Input: part model. Units: mm. Frame: model coordinates. Face numbers are marked on the shaded views. A direction names the side the tool comes from. Coordinates: 2 decimals unless noted, no trailing zeros. Order: outer loops, then holes, each group sorted by start corner. A loop starts at its lowest first (then second) coordinate and runs counter-clockwise, first axis right, second up. Notation, with made-up numbers: (56, 64.5) -> (109, 64.5) arc R34 ccw to (109, 94.5) -> close; hole circle Ø1 at (-8.75, -24.5). An arc over 180 degrees is marked (long way). Use one line per item in the form item = value. Start each with the question number.
1) Ray query, line 1 along X through (y, z) = (12.9, -96.25); line 2 along Z through (x, y) = (61.5, 12.5); line 3 along X through (y, z) = (12, -1). Return the intervals inside material, ascending.
2) Section query C-C on z = -77.5. Output: boundary loops of the cut face in (x, y), then the cut area to 3 significant figures.
3) Section query A-A on x = 36. Output: boundary loops of the cut face in (y, z), then the cut area to 3 significant figures.
4) Section query B-B on y = 15.5. Output: boundary loops of the cut face in (x, z), then the cut area to 3 significant figures.
5) Pin query (flat end, axial travel): pin 1 (1.2 mm diameter, centred on x = 59.5, y = 22.9, fed in from +Z); pin 2 (4 mm diameter, centred on y = 29, z = -70.5, fed in from -X); pin 3 (5 mm diameter, centred on x = 15, z = -66, fed in from +Y). Return the tip coordinate at first contact, or that it passes through.
6) Access query for the marked faces 1 and 2. Directions: +Z, -Z, +X, -X, +Y, -Y. A direction counts if a zero-diameter tool reaches every point of the face in a straight line with its end or side. Return the directions, or none.
from build123d import *

# Parameters (mm, degrees)
SKETCH1_W            = 70
SKETCH1_H            = 50
BOSS_EXTRUDE1_DEPTH  = 7.5
SKETCH2_W            = 70
SKETCH2_H            = 5
BOSS_EXTRUDE2_DEPTH  = 25
SKETCH3_R            = 1
SKETCH3_W            = 42
SKETCH3_H            = 21
CUT_EXTRUDE1_DEPTH   = 30
SKETCH27_W           = 5
SKETCH27_H           = 25
BOSS_EXTRUDE18_DEPTH = 45


with BuildPart() as part:
    # Sketch1 → Boss-Extrude1 (new body)
    with BuildSketch(Plane(origin=(0, 0, 0), x_dir=(1, 0, 0), z_dir=(0, 1, 0))):
        with Locations((35, 25)):
            Rectangle(SKETCH1_W, SKETCH1_H)
    boss_extrude1 = extrude(amount=BOSS_EXTRUDE1_DEPTH)

    # Sketch2 → Boss-Extrude2 (add)
    with BuildSketch(Plane(origin=(0, 7.5, 0), x_dir=(1, 0, 0), z_dir=(0, 1, 0))):
        with Locations((35, 2.5)):
            Rectangle(SKETCH2_W, SKETCH2_H)
    boss_extrude2 = extrude(amount=BOSS_EXTRUDE2_DEPTH)

    # Sketch3 → Cut-Extrude1 (cut)
    with BuildSketch(Plane.XY):
        with Locations((9.720773398, 22.9)):
            Circle(SKETCH3_R)
        with Locations((9.720773398, 12.9)):
            Circle(SKETCH3_R)
        with Locations((59.5, 12.9)):
            Circle(SKETCH3_R)
        with Locations((59.5, 22.9)):
            Circle(SKETCH3_R)
        with Locations((34.5, 18)):
            Rectangle(SKETCH3_W, SKETCH3_H)
    cut_extrude1 = extrude(amount=-CUT_EXTRUDE1_DEPTH, mode=Mode.SUBTRACT)

    # Sketch27 → Boss-Extrude18 (add)
    with BuildSketch(Plane(origin=(0, 0, -5), x_dir=(-1, 0, 0), z_dir=(0, 0, -1))):
        with Locations((-67.5, 20)):
            Rectangle(SKETCH27_W, SKETCH27_H)
    boss_extrude18 = extrude(amount=BOSS_EXTRUDE18_DEPTH)

    # Mirror1: Boss-Extrude1, Boss-Extrude2, Cut-Extrude1, Boss-Extrude18 across plane
    add(boss_extrude1.mirror(Plane(origin=(0, 0, -50), x_dir=(1, 0, 0), z_dir=(0, 0, -1))))
    add(boss_extrude2.mirror(Plane(origin=(0, 0, -50), x_dir=(1, 0, 0), z_dir=(0, 0, -1))))
    add(cut_extrude1.mirror(Plane(origin=(0, 0, -50), x_dir=(1, 0, 0), z_dir=(0, 0, -1))), mode=Mode.SUBTRACT)
    add(boss_extrude18.mirror(Plane(origin=(0, 0, -50), x_dir=(1, 0, 0), z_dir=(0, 0, -1))))


solid = part.part
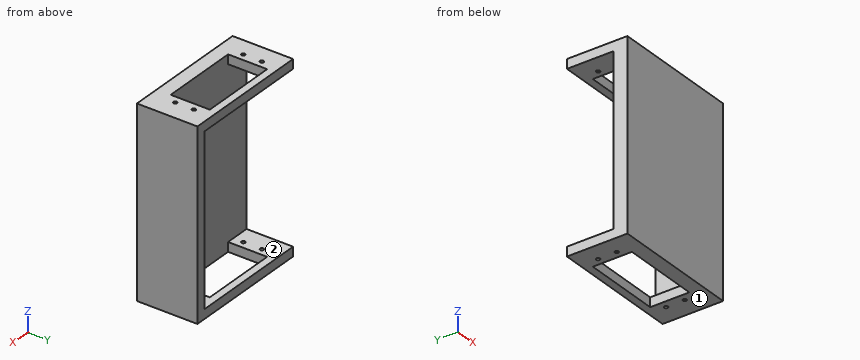
Answers below:
q1.line_1 = 0 to 8.72, 10.72 to 13.5, 55.5 to 58.5, 60.5 to 70
q1.line_2 = -100 to -95, -5 to 0
q1.line_3 = 0 to 9.28, 10.16 to 13.5, 55.5 to 59.06, 59.94 to 70
q2.outline = (0, 0) -> (70, 0) -> (70, 32.5) -> (65, 32.5) -> (65, 7.5) -> (0, 7.5) -> close
q2.area = 650 mm^2
q3.outline = (0, -100) -> (7.5, -100) -> (7.5, 0) -> (0, 0) -> close; (28.5, -100) -> (32.5, -100) -> (32.5, -95) -> (28.5, -95) -> close; (28.5, -5) -> (32.5, -5) -> (32.5, 0) -> (28.5, 0) -> close
q3.area = 790 mm^2
q4.outline = (0, -100) -> (13.5, -100) -> (13.5, -95) -> (0, -95) -> close; (0, -5) -> (13.5, -5) -> (13.5, 0) -> (0, 0) -> close; (55.5, -100) -> (70, -100) -> (70, 0) -> (55.5, 0) -> (55.5, -5) -> (65, -5) -> (65, -95) -> (55.5, -95) -> close
q4.area = 730 mm^2
q5.pin_1 = through
q5.pin_2 = 65
q5.pin_3 = 7.5
q6.face_1 = -Z, +X, -X, +Y, -Y
q6.face_2 = -X, +Y
